```python
from build123d import *

# Parameters (mm, degrees)
F2_DEPTH = 12.7
F1_R     = 69.346694
F3_DEPTH = 12.7
F4_COUNT = 10


with BuildPart() as f2:
    # F0 (on Front) → F2 (new body)
    with BuildSketch(Plane.XZ):
        with BuildLine():
            Line((22.197887, 39.416865), (50.918356, 39.377556))
            ThreePointArc((50.918356, 39.377556), (48.579291, 50.769767), (41.914459, 60.300438))
            Line((41.914459, 60.300438), (31.243502, 60.300438))
            ThreePointArc((31.243502, 60.300438), (24.563893, 50.792859), (22.197887, 39.416865))
        make_face()
    extrude(amount=F2_DEPTH)

    # F1 (on Front) → F3 (join)
    with BuildSketch(Plane.XZ):
        with Locations((37.202269, -25.696449)):
            Circle(F1_R)
    extrude(amount=F3_DEPTH)

    # F4: F2 ×10 about axis
    f4_axis = Axis((37.202269, 0, -25.696449), (0, 1, 0))


with BuildPart() as f2_1:
    add(f2.part)
    for i in range(1, F4_COUNT):
        add(f2.part.rotate(f4_axis, i * 360 / F4_COUNT))


solid = f2_1.part
```
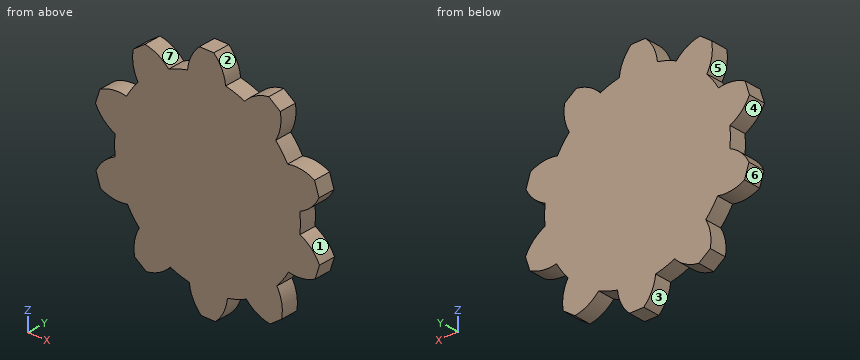
Work out the finished part from the listing and answer in its coordinate system (mm). Face numbers are marked on the shaded views. A direction names the side the tool comes from. Give positions to 0.01 mm unless a question says otherwise; leave off trailing zeros. Loops run counter-clockwise (first coordinate to the right, second up) from the corner with the lowest first, then second, coordinate; pieces in that order, holes last. Notation, with made-up numbers: (80, 64.5) -> (98, 64.5) arc R36 cw to (98, 102.5) -> close; hole circle Ø5 at (80.5, -5). An arc over 180 degrees is marked (long way). One line per question, with ' | ' between items. Start each with the question number.
1) Straight lines are drawn through the part: L1, parallel to X at y = -7, z = -25.5; L2, parallel to Z at x = -34, y = -3.5; L3, parallel to X at y = -1.75, z = -3. For each, find the intervals that lie inside material, in ascending order.
2) Section B-B, the plane x = 15 is taken. Determine the outline of the cut face in (y, z).
3) Section A-A, the plane z = 30 is taken. Determine the outline of the cut face in (x, y), then the cut area to 3 significant figures.
4) Determine the mould class of the marked faces 5, 6 and 7 for opening direction Z: +Z half, -Z half, draft (parallel to the pull), parting line (faces both ways), or undercut.
5) For the marked faces 1, 2, 3 and 4, determine the directions among +Z, -Z, +X, -X, +Y, -Y from which every point of the face is accessible in a straight line to the end or side of a thin tool.
6) Each of these flat-tipped pins is pushed along its axis until it touches: pin 1 (4 mm diameter, centred on x = -9.5, y = -9.5, fed in from +Z); pin 2 (2 mm diameter, centred on x = 9.5, y = -2.5, fed in from -Z); pin 3 (6 mm diameter, centred on x = -26.5, y = -3, fed in from -Z). Where does it stop, or does it pass through?
Resolved:
1) L1: -32.14 to 106.55 | L2: -61.03 to -34.96, -17.86 to 8.5 | L3: -45.85 to 120.25
2) outline: (-12.7, -91.39) -> (0, -91.39) -> (0, 40) -> (-12.7, 40) -> close
3) outline: (-18.23, -12.7) -> (91.46, -12.7) -> (91.46, 0) -> (-18.23, 0) -> close | area: 1,390 mm2
4) face 5: undercut | face 6: -Z half | face 7: +Z half
5) face 1: +X, +Y, -Y | face 2: +Z, +Y, -Y | face 3: -Z, +Y, -Y | face 4: -X, +Y, -Y
6) pin 1: z = 46.65 | pin 2: z = -90.25 | pin 3: z = -61.48
